Can you work these out from the model? Positions are in its coordinate system, mm. A direction names the side the tool comes from. Coordinates: 2 decimals unless noted, no trailing zeros. Order: outer loops, then holes, each group sorted by start corner. A loop starts at its lowest first (then second) coordinate and runs counter-clockwise, first axis right, second up. Notation, with made-up numbers: (75.5, 70.25) -> (134.5, 70.25) arc R25 cw to (134.5, 86.25) -> close; hole circle Ø11 at (34, 30.25). An arc over 180 degrees is marked (long way). Return JSON: item names as keys, results as strings. Group by question number.
1) For pin 1 (4 mm diameter, centred on x = 16.5, z = -59.5, fed in from +Y); pin 2 (21 mm diameter, centred on x = 30, z = 80.5, fed in from +Y); pin 3 (2 mm diameter, centred on x = 36, z = -98, fed in from +Y), each with a flat end and sliding along its axis, tell me the tip position at first contact or that it passes through.
2) If I drill on probe 1 along X at (y, z) = (4.15, -21); probe 2 along X at (y, z) = (3.5, -98); probe 3 along X at (y, z) = (10.5, 37), over which ranges is the centre line in solid material (lowest first)? Write a range as from..to.
3) For faces 1 (the flat face through (44.5, 10, 5)), 2 (the cylindrical face through (-46.07, 5.22, 103.5)), 3 (the cylindrical face through (-37.71, 3.78, -98.38)), 4 (the flat face through (-44.5, 10, 3)), 5 (the flat face through (1, 9, 100)), which set-ups out of +Z, -Z, +X, -X, +Y, -Y let a thin tool reach every point of the face, with its end or its side?
4) Thinking about a two-plate mould opening in Z: for faces 6 (the flat face through (-1, 9, 102)), 7 (the cylindrical face through (-46, 5.22, -103.57)), 8 (the flat face through (43, 12.4, 6)), 9 (the cylindrical face through (-32.034, 5.493, -46.521)), which applies, +Z half, -Z half, draft (parallel to the pull), parting line (faces both ways), or undercut?
5) If we section it at A-A, the plane z = -83: Please give me the cut outline in (x, y).
from build123d import *

# Parameters (mm, degrees)
BOSS_EXTRUDE1_DEPTH             = 3
BOSS_EXTRUDE2_DEPTH             = 4.5
SKETCH3_R                       = 4
SKETCH3_R_2                     = 1.4
SKETCH3_R_3                     = 12.15
BOSS_EXTRUDE3_DEPTH             = 3
CUT_EXTRUDE3_REACH              = 117.4
SKETCH6_R                       = 1.75
BOSS_EXTRUDE5_DEPTH             = 4.9
BOSS_EXTRUDE5_DIRECTION_2_REACH = 117.488
FILLET3_R                       = 3
BOSS_EXTRUDE6_DEPTH             = 0.9
FILLET4_R                       = 0.9
CHAMFER4_SIZE                   = 1.5
FILLET6_R                       = 2
FILLET7_R                       = 3


with BuildPart() as part:
    # Sketch1 → Boss-Extrude1 (new body)
    with BuildSketch(Plane(origin=(0, 0, 0), x_dir=(1, 0, 0), z_dir=(0, 1, 0))):
        with BuildLine():
            Line((-42.5, -105), (42.5, -105))
            ThreePointArc((42.5, -105), (46.035533906, -103.535533906), (47.5, -100))
            Line((47.5, -100), (47.5, 100))
            ThreePointArc((47.5, 100), (46.035533906, 103.535533906), (42.5, 105))
            Line((42.5, 105), (-42.5, 105))
            ThreePointArc((-42.5, 105), (-46.035533906, 103.535533906), (-47.5, 100))
            Line((-47.5, 100), (-47.5, -100))
            ThreePointArc((-47.5, -100), (-46.035533906, -103.535533906), (-42.5, -105))
        make_face()
    extrude(amount=BOSS_EXTRUDE1_DEPTH)

    # Sketch2 → Boss-Extrude2 (add)
    with BuildSketch(Plane(origin=(0, 3, 0), x_dir=(1, 0, 0), z_dir=(0, 1, 0))):
        with BuildLine():
            Line((42.5, 105), (-42.5, 105))
            ThreePointArc((-42.5, 105), (-46.035533906, 103.535533906), (-47.5, 100))
            Line((-47.5, 100), (-47.5, -100))
            ThreePointArc((-47.5, -100), (-46.035533906, -103.535533906), (-42.5, -105))
            Line((-42.5, -105), (42.5, -105))
            ThreePointArc((42.5, -105), (46.035533906, -103.535533906), (47.5, -100))
            Line((47.5, -100), (47.5, 100))
            ThreePointArc((47.5, 100), (46.035533906, 103.535533906), (42.5, 105))
        make_face()
        with BuildLine():
            Line((42.5, 102), (-42.5, 102))
            ThreePointArc((-42.5, 102), (-43.914213562, 101.414213562), (-44.5, 100))
            Line((-44.5, 100), (-44.5, -100))
            ThreePointArc((-44.5, -100), (-43.914213562, -101.414213562), (-42.5, -102))
            Line((-42.5, -102), (42.5, -102))
            ThreePointArc((42.5, -102), (43.914213562, -101.414213562), (44.5, -100))
            Line((44.5, -100), (44.5, 100))
            ThreePointArc((44.5, 100), (43.914213562, 101.414213562), (42.5, 102))
        make_face(mode=Mode.SUBTRACT)
    extrude(amount=BOSS_EXTRUDE2_DEPTH)

    # Sketch3 → Boss-Extrude3 (add)
    # profile 1 of 8: a face of its own
    with BuildSketch(Plane(origin=(0, 3, 0), x_dir=(1, 0, 0), z_dir=(0, 1, 0))):
        with Locations(Location((-36, 46, 0), (0, 0, 270))):
            Circle(SKETCH3_R)
        with Locations(Location((-36, 46, 0), (0, 0, 270))):
            Circle(SKETCH3_R_2, mode=Mode.SUBTRACT)
    # profile 2 of 8: a face of its own
    with BuildSketch(Plane(origin=(0, 3, 0), x_dir=(1, 0, 0), z_dir=(0, 1, 0))):
        with Locations(Location((36, 46, 0), (0, 0, 90))):
            Circle(SKETCH3_R)
        with Locations(Location((36, 46, 0), (0, 0, 90))):
            Circle(SKETCH3_R_2, mode=Mode.SUBTRACT)
    # profile 3 of 8: a face of its own
    with BuildSketch(Plane(origin=(0, 3, 0), x_dir=(1, 0, 0), z_dir=(0, 1, 0))):
        with BuildLine():
            Line((-15, -91.126617032), (-15, -102))
            Line((-15, -102), (-44.5, -102))
            Line((-44.5, -102), (-44.5, -73.85))
            Line((-44.5, -73.85), (-30, -73.85))
            ThreePointArc((-30, -73.85), (-18.560140997, -79.06762234), (-15, -91.126617032))
        make_face()
        with Locations(Location((-30, -89, 0), (0, 0, 270))):
            Circle(SKETCH3_R_3, mode=Mode.SUBTRACT)
    # profile 4 of 8: a face of its own
    with BuildSketch(Plane(origin=(0, 3, 0), x_dir=(1, 0, 0), z_dir=(0, 1, 0))):
        with BuildLine():
            Line((-40, 98), (-40, 102))
            Line((-40, 102), (-32, 102))
            Line((-32, 102), (-32, 98))
            ThreePointArc((-32, 98), (-36, 94), (-40, 98))
        make_face()
        with Locations(Location((-36, 98, 0), (0, 0, 270))):
            Circle(SKETCH3_R_2, mode=Mode.SUBTRACT)
    # profile 5 of 8: a face of its own
    with BuildSketch(Plane(origin=(0, 3, 0), x_dir=(1, 0, 0), z_dir=(0, 1, 0))):
        with BuildLine():
            Line((32, 102), (32, 98))
            ThreePointArc((32, 98), (36, 94), (40, 98))
            Line((40, 98), (40, 102))
            Line((40, 102), (32, 102))
        make_face()
        with Locations(Location((36, 98, 0), (0, 0, 90))):
            Circle(SKETCH3_R_2, mode=Mode.SUBTRACT)
    # profile 6 of 8: a face of its own
    with BuildSketch(Plane(origin=(0, 3, 0), x_dir=(1, 0, 0), z_dir=(0, 1, 0))):
        with BuildLine():
            Line((-30, 36.15), (-44.5, 36.15))
            Line((-44.5, 36.15), (-44.5, 5.85))
            Line((-44.5, 5.85), (-30, 5.85))
            ThreePointArc((-30, 5.85), (-14.85, 21), (-30, 36.15))
        make_face()
        with Locations(Location((-30, 21, 0), (0, 0, 270))):
            Circle(SKETCH3_R_3, mode=Mode.SUBTRACT)
    # profile 7 of 8: a face of its own
    with BuildSketch(Plane(origin=(0, 3, 0), x_dir=(1, 0, 0), z_dir=(0, 1, 0))):
        with BuildLine():
            Line((44.5, 5.85), (30, 5.85))
            ThreePointArc((30, 5.85), (14.85, 21), (30, 36.15))
            Line((30, 36.15), (44.5, 36.15))
            Line((44.5, 36.15), (44.5, 5.85))
        make_face()
        with Locations(Location((30, 21, 0), (0, 0, 90))):
            Circle(SKETCH3_R_3, mode=Mode.SUBTRACT)
    # profile 8 of 8: a face of its own
    with BuildSketch(Plane(origin=(0, 3, 0), x_dir=(1, 0, 0), z_dir=(0, 1, 0))):
        with BuildLine():
            Line((15, -102), (44.5, -102))
            Line((44.5, -102), (44.5, -73.85))
            Line((44.5, -73.85), (30, -73.85))
            ThreePointArc((30, -73.85), (18.560140997, -79.06762234), (15, -91.126617032))
            Line((15, -91.126617032), (15, -102))
        make_face()
        with Locations(Location((30, -89, 0), (0, 0, 90))):
            Circle(SKETCH3_R_3, mode=Mode.SUBTRACT)
    extrude(amount=BOSS_EXTRUDE3_DEPTH)

    # Sketch6 → Cut-Extrude3 (cut, up to next)
    with BuildSketch(Plane(origin=(0, 6, 0), x_dir=(1, 0, 0), z_dir=(0, 1, 0)), mode=Mode.PRIVATE) as cut_extrude3_sk1:
        with Locations(Location((-36, 98, 0), (0, 0, 270))):
            Circle(SKETCH6_R)
    cut_extrude3_tool1 = extrude(cut_extrude3_sk1.sketch, amount=-CUT_EXTRUDE3_REACH, mode=Mode.PRIVATE) & part.part
    # Sketch6 → Cut-Extrude3 (cut, up to next)
    with BuildSketch(Plane(origin=(0, 6, 0), x_dir=(1, 0, 0), z_dir=(0, 1, 0)), mode=Mode.PRIVATE) as cut_extrude3_sk2:
        with Locations(Location((36, 98, 0), (0, 0, 270))):
            Circle(SKETCH6_R)
    cut_extrude3_tool2 = extrude(cut_extrude3_sk2.sketch, amount=-CUT_EXTRUDE3_REACH, mode=Mode.PRIVATE) & part.part
    # Sketch6 → Cut-Extrude3 (cut, up to next)
    with BuildSketch(Plane(origin=(0, 6, 0), x_dir=(1, 0, 0), z_dir=(0, 1, 0)), mode=Mode.PRIVATE) as cut_extrude3_sk3:
        with Locations(Location((-36, 46, 0), (0, 0, 270))):
            Circle(SKETCH6_R)
    cut_extrude3_tool3 = extrude(cut_extrude3_sk3.sketch, amount=-CUT_EXTRUDE3_REACH, mode=Mode.PRIVATE) & part.part
    # Sketch6 → Cut-Extrude3 (cut, up to next)
    with BuildSketch(Plane(origin=(0, 6, 0), x_dir=(1, 0, 0), z_dir=(0, 1, 0)), mode=Mode.PRIVATE) as cut_extrude3_sk4:
        with Locations(Location((36, 46, 0), (0, 0, 270))):
            Circle(SKETCH6_R)
    cut_extrude3_tool4 = extrude(cut_extrude3_sk4.sketch, amount=-CUT_EXTRUDE3_REACH, mode=Mode.PRIVATE) & part.part
    add(cut_extrude3_tool1.solids().sort_by_distance((-36, 6, -98))[0], mode=Mode.SUBTRACT)
    add(cut_extrude3_tool2.solids().sort_by_distance((36, 6, -98))[0], mode=Mode.SUBTRACT)
    add(cut_extrude3_tool3.solids().sort_by_distance((-36, 6, -46))[0], mode=Mode.SUBTRACT)
    add(cut_extrude3_tool4.solids().sort_by_distance((36, 6, -46))[0], mode=Mode.SUBTRACT)

    # Sketch5 → Boss-Extrude5 (add)
    with BuildSketch(Plane(origin=(0, 7.5, 0), x_dir=(1, 0, 0), z_dir=(0, 1, 0))):
        with BuildLine():
            Line((-42.5, -102), (42.5, -102))
            ThreePointArc((42.5, -102), (43.914213562, -101.414213562), (44.5, -100))
            Line((44.5, -100), (44.5, 92))
            Line((44.5, 92), (42.5, 92))
            Line((42.5, 92), (42.5, -100))
            Line((42.5, -100), (-42.5, -100))
            Line((-42.5, -100), (-42.5, 92))
            Line((-42.5, 92), (-44.5, 92))
            Line((-44.5, 92), (-44.5, -100))
            ThreePointArc((-44.5, -100), (-43.914213562, -101.414213562), (-42.5, -102))
        make_face()
    extrude(amount=BOSS_EXTRUDE5_DEPTH)

    # Sketch5 → Boss-Extrude5 direction 2 (add, up to next)
    with BuildSketch(Plane(origin=(0, 7.5, 0), x_dir=(1, 0, 0), z_dir=(0, 1, 0)), mode=Mode.PRIVATE) as boss_extrude5_direction_2_sk1:
        with BuildLine():
            Line((-42.5, -102), (42.5, -102))
            ThreePointArc((42.5, -102), (43.914213562, -101.414213562), (44.5, -100))
            Line((44.5, -100), (44.5, 92))
            Line((44.5, 92), (42.5, 92))
            Line((42.5, 92), (42.5, -100))
            Line((42.5, -100), (-42.5, -100))
            Line((-42.5, -100), (-42.5, 92))
            Line((-42.5, 92), (-44.5, 92))
            Line((-44.5, 92), (-44.5, -100))
            ThreePointArc((-44.5, -100), (-43.914213562, -101.414213562), (-42.5, -102))
        make_face()
    boss_extrude5_direction_2_tool1 = extrude(boss_extrude5_direction_2_sk1.sketch, amount=-BOSS_EXTRUDE5_DIRECTION_2_REACH, mode=Mode.PRIVATE) - part.part
    add(boss_extrude5_direction_2_tool1.solids().sort_by_distance((-43.763288, 7.5, 101.263288))[0])

    # Fillet3
    fillet3_edges = [part.edges().sort_by_distance(p)[0] for p in [
        (43.5, 12.4, -92),
        (-43.5, 12.4, -92),
    ]]
    fillet(fillet3_edges, radius=FILLET3_R)

    # Sketch8 → Boss-Extrude6 (add)
    with BuildSketch(Plane.XY.offset(102)):
        with BuildLine():
            Line((-25, 11.4), (25, 11.4))
            ThreePointArc((25, 11.4), (25.9, 10.5), (25, 9.6))
            Line((25, 9.6), (-25, 9.6))
            ThreePointArc((-25, 9.6), (-25.9, 10.5), (-25, 11.4))
        make_face()
    extrude(amount=BOSS_EXTRUDE6_DEPTH)

    # Fillet4
    fillet4_edges = [part.edges().sort_by_distance(p)[0] for p in [
        (25.9, 10.5, 102.9),
        (0, 9.6, 102.9),
        (-25.9, 10.5, 102.9),
        (0, 11.4, 102.9),
    ]]
    fillet(fillet4_edges, radius=FILLET4_R - 0.0001)  # a hair under: the kernel refuses the full size

    # Chamfer4
    chamfer4_edges = [part.edges().sort_by_distance(p)[0] for p in [
        (36, 0, -99.75),
        (-36, 0, -47.75),
        (36, 0, -47.75),
        (-36, 0, -99.75),
    ]]
    chamfer(chamfer4_edges, length=CHAMFER4_SIZE)

    # Fillet6
    fillet6_edges = [part.edges().sort_by_distance(p)[0] for p in [
        (36, 3, -94),
        (40, 3, -100),
        (32, 3, -100),
        (-36, 3, -50),
        (-32, 3, -100),
        (-40, 3, -100),
        (-36, 3, -94),
        (36, 3, -42),
    ]]
    fillet(fillet6_edges, radius=FILLET6_R)

    # Fillet7
    fillet7_edges = [part.edges().sort_by_distance(p)[0] for p in [
        (0, 0, -105),
        (46.035533906, 0, -103.535533906),
        (47.5, 0, 0),
        (46.035533906, 0, 103.535533906),
        (0, 0, 105),
        (-46.035533906, 0, 103.535533906),
        (-47.5, 0, 0),
        (-46.035533906, 0, -103.535533906),
    ]]
    fillet(fillet7_edges, radius=FILLET7_R)


solid = part.part
Result sheet:
{
 "1": {"pin 1": "stops at y = 3", "pin 2": "stops at y = 6", "pin 3": "passes through"},
 "2": {"probe 1": "x = -47.5..-42.15, -17.85..-14.85, 14.85..17.85, 42.15..47.5", "probe 2": "x = -47.5..-44.5, -40.68..-37.75, -34.25..-31.32, 31.32..34.25, 37.75..40.68, 44.5..47.5", "probe 3": "x = -44.5..-42.5, 42.5..44.5"},
 "3": {"face 1": "+Z, -Z, +X, +Y", "face 2": "+Z, -X, +Y, -Y", "face 3": "+Y, -Y", "face 4": "+Z, -Z, -X, +Y", "face 5": "+Y"},
 "4": {"face 6": "+Z half", "face 7": "-Z half", "face 8": "draft", "face 9": "undercut"},
 "5": {"outline": "(-47.5, 3) arc R3 ccw to (-44.5, 0) -> (44.5, 0) arc R3 ccw to (47.5, 3) -> (47.5, 7.5) -> (44.5, 7.5) -> (44.5, 12.4) -> (42.5, 12.4) -> (42.5, 3) -> (-42.5, 3) -> (-42.5, 12.4) -> (-44.5, 12.4) -> (-44.5, 7.5) -> (-47.5, 7.5) -> close"}
}
